Check sheet for the modelled part. Datum: model origin and axes. Units: mm. Face numbers are marked on the shaded views. Coordinates: 2 decimals unless noted, no trailing zeros. Loops run counter-clockwise (first coordinate to the right, second up) from the corner with the lowest first, then second, coordinate; pieces in that order, holes last. Notation, with made-up numbers: (67, 59) - (72, 59) arc R27 cw to (72, 78) - close; hole circle Ø9 at (32.25, 6.25). An arc over 180 degrees is marked (long way). Use a Markdown table: item, result. Add a question column.
1) Go/stop test with flat-tipped pins: P1, Ø1.5, axis at x = -47.5, z = 2, coming from the -Y side; P2, Ø4, axis at x = -33, y = -17.5, coming from the -Z side. Record where each tip stops, or that it passes through.
2) Sectioned sample at D-D, the plane x = -45. Enter the section's corners in (y, z).
3) Sectioned sample at C-C, the plane x = -62.5. Enter the section's corners in (y, z), then the cut area to 3 significant figures.
4) Sectioned sample at B-B, the plane y = -7. Enter the section's corners in (x, z).
5) Sectioned sample at A-A, the plane z = 1.15. Enter the section's corners in (x, y), then the cut area to 3 significant figures.
6) Thickness scan on line 1 (Y direction, x = -36, z = 3); line 2 (X direction, y = -11, z = 1.95); line 3 (X direction, y = -28, z = 0.5). Record the ranges inside material, lowest first.
7) Draft check along X on the marked faces 1 and 2. Enter one of: pulls with the +X half, pulls with the -X half, needs draft (parallel to the pull), parting line crosses it, or undercut.
from build123d import *

# Parameters (mm, degrees)
BOSS_EXTRUDE1_DEPTH = 5
SKETCH2_R           = 5
CUT_EXTRUDE1_DEPTH  = 5


with BuildPart() as part:
    # Sketch1 → Boss-Extrude1 (new body)
    with BuildSketch(Plane.XY):
        Polygon((-73.283312465, -1.804635762), (26.716687535, -1.804635762), (26.716687535, -41.804635762), (11.716687535, -41.804635762), (11.716687535, -16.804635762), (-73.283312465, -16.804635762), align=None)
    extrude(amount=BOSS_EXTRUDE1_DEPTH)

    # Sketch2 → Cut-Extrude1 (cut)
    with BuildSketch(Plane.XY.offset(5)):
        with Locations((19.216687535, -34.304635762)):
            Circle(SKETCH2_R)
        with BuildLine():
            ThreePointArc((19.216687535, -41.804635762), (13.913386676, -39.60793662), (11.716687535, -34.304635762))
            Line((11.716687535, -34.304635762), (11.716687535, -41.804635762))
            Line((11.716687535, -41.804635762), (19.216687535, -41.804635762))
        make_face()
        with BuildLine():
            Line((26.716687535, -41.804635762), (26.716687535, -34.304635762))
            ThreePointArc((26.716687535, -34.304635762), (24.519988394, -39.60793662), (19.216687535, -41.804635762))
            Line((19.216687535, -41.804635762), (26.716687535, -41.804635762))
        make_face()
        with Locations((-65.783312465, -9.304635762)):
            Circle(SKETCH2_R)
        with BuildLine():
            Line((-65.783312465, -1.804635762), (-73.283312465, -1.804635762))
            Line((-73.283312465, -1.804635762), (-73.283312465, -9.304635859))
            ThreePointArc((-73.283312465, -9.304635859), (-71.086613359, -4.001334937), (-65.783312465, -1.804635762))
        make_face()
        with BuildLine():
            ThreePointArc((-65.783312465, -16.804635762), (-71.086613289, -14.607936655), (-73.283312465, -9.304635859))
            Line((-73.283312465, -9.304635859), (-73.283312465, -16.804635762))
            Line((-73.283312465, -16.804635762), (-65.783312465, -16.804635762))
        make_face()
    extrude(amount=-CUT_EXTRUDE1_DEPTH, mode=Mode.SUBTRACT)


solid = part.part
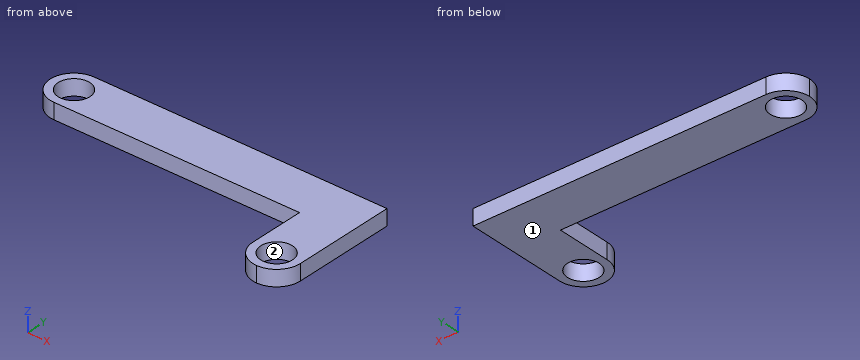
Solved:
| question | item | result |
|---|---|---|
| 1 | P1 | stops at y = -16.8 |
| 1 | P2 | stops at z = 0 |
| 2 | outline | (-16.8, 0) - (-1.8, 0) - (-1.8, 5) - (-16.8, 5) - close |
| 3 | outline | (-16.8, 0) - (-13.08, 0) - (-13.08, 5) - (-16.8, 5) - close; (-5.53, 0) - (-1.8, 0) - (-1.8, 5) - (-5.53, 5) - close |
| 3 | area | 37.3 mm2 |
| 4 | outline | (-72.92, 0) - (-70.22, 0) - (-70.22, 5) - (-72.92, 5) - close; (-61.35, 0) - (26.72, 0) - (26.72, 5) - (-61.35, 5) - close |
| 5 | outline | (-65.78, -16.8) - (11.72, -16.8) - (11.72, -34.3) arc R7.5 ccw to (26.72, -34.3) - (26.72, -1.8) - (-65.78, -1.8) arc R7.5 ccw to start; hole circle Ø10 at (-65.78, -9.3); hole circle Ø10 at (19.22, -34.3) |
| 5 | area | 1,670 mm2 |
| 6 | line 1 | y = -16.8 to -1.8 |
| 6 | line 2 | x = -73.09 to -70.49, -61.08 to 26.72 |
| 6 | line 3 | x = 11.72 to 26.72 |
| 7 | face 1 | needs draft |
| 7 | face 2 | undercut |
